CAD build for the part. Positions are in the model's coordinates, mm. A direction names the side the tool comes from. Coordinates: 2 decimals unless noted, no trailing zeros. Order: outer loops, then holes, each group sorted by start corner. A loop starts at its lowest first (then second) coordinate and runs counter-clockwise, first axis right, second up. Notation, with made-up numbers: M 43,83.5 L 62,83.5 A18 cw 62,104.5 Z; hole C 1.5,-7 d6. An arc over 180 degrees is marked long. Write item = value, one per line. Start each with the question number.
Autodesk Inventor part; units mm, degrees
ref_plane "YZ Plane" through (0, 0, 0) normal (1, 0, 0) x (0, 1, 0)
ref_plane "XZ Plane" through (0, 0, 0) normal (0, 1, 0) x (-1, 0, 0)
ref_plane "XY Plane" through (0, 0, 0) normal (0, 0, 1) x (1, 0, 0)
sketch "Sketch1" plane through (0, 0, 0) normal (0, 0, 1) x (1, 0, 0)
  line L0 (0, 0) -> (-132, 0)
  line L1 (-132, 0) -> (-132, -5)
  line L2 (-132, -5) -> (0, -5)
  line L3 (0, -5) -> (0, 0)
  dimension "d0" = 5
  dimension "d1" = 132
extrude "Extrusion1" add sketch "Sketch1" along normal blind 30
sketch "Sketch2" plane through (-132, 0, 0) normal (0, 1, 0) x (1, 0, 0)
  line L0 (0, -30) -> (132, -30)
  line L1 (0, -30) -> (5, -30)
  line L2 (5, -30) -> (5, -15)
  line L3 (5, -15) -> (0, -15)
  line L4 (0, -15) -> (0, -30)
  line L5 (132, -30) -> (127, -30)
  line L6 (127, -30) -> (127, -15)
  line L7 (127, -15) -> (132, -15)
  line L8 (132, -15) -> (132, -30)
  line L9 (0, 0) -> (0, -30)
  line L10 (132, 0) -> (132, -30)
  line L11 (0, 0) -> (132, 0)
  line L12 (132, 0) -> (132, 0)
  line L13 (132, 0) -> (0, 0)
  line L14 (0, 0) -> (0, 0)
  line L15 (0, 0) -> (5, 0)
  line L16 (5, 0) -> (5, -5)
  line L17 (5, -5) -> (0, -5)
  line L18 (0, -5) -> (0, 0)
  line L19 (132, 0) -> (127, 0)
  line L20 (127, 0) -> (127, -5)
  line L21 (127, -5) -> (132, -5)
  line L22 (132, -5) -> (132, 0)
  point P0 (5, -30)
  point P1 (5, 0)
  point P2 (127, 0)
  dimension "d4" = 5
  dimension "d5" = 15
  dimension "d6" = 15
  dimension "d7" = 5
  dimension "d8" = 0
  dimension "d11" = 5
  dimension "d12" = 5
  dimension "d13" = 5
  dimension "d14" = 10
extrude "Extrusion2" cut sketch "Sketch2" against normal blind 10 contours L4 L3 L2 L0 | L6 L7 L8 L0 | L9 L11 L16 L17 | L21 L20 L11 L10
properties part number "FANsuport"
1. Mould opens along X. For faces 1 (the flat face through (-127, -2, 2)), 2 (the flat face through (-5, -2, 23)), 3 (the flat face through (-129, -2, 15)) say: released by +X, released by -X, zero draft, split by the parting line, or undercut.
2. Slice it at B-B (z = 18). Write the cut outline in (x, y), plus the area to 3 significant figures.
3. 3-axis set-ups, long thin cutter, end or side, ignore diameter. For faces 4 (the flat face through (-3, -2, 15)), 5 (the flat face through (-67, -2, 30)), 6 (the flat face through (-3, -2, 5)), 7 (the flat face through (-129, -2, 5)), 8 (the flat face through (-127, -2, 23)): which of +Z, -Z, +X, -X, +Y, -Y reach the whole face in a straight line?
4. Probe L1, parallel to X at y = -0.9, z = 4.75. List the from-to ranges inside material, lowest first.
5. Flat gauge pins, fed straight in: pin 1 (3 mm diameter, centred on x = -38, z = 5.5, fed in from +Y); pin 2 (1.5 mm diameter, centred on x = -130, y = -3.5, fed in from -Z); pin 3 (1.5 mm diameter, centred on y = -2.5, z = 24.5, fed in from +X); pin 4 (1.5 mm diameter, centred on x = -129.5, y = -3, fed in from +Z). Where does each tip first touch, or does it go through?
6. Slice it at A-A (y = -3.95). Write the cut outline in (x, z).
Calculated:
q1.face_1 = released by -X
q1.face_2 = released by +X
q1.face_3 = zero draft
q2.outline = M -127,-5 L -5,-5 L -5,0 L -127,0 Z
q2.area = 610 mm²
q3.face_4 = +Z, +X, +Y, -Y
q3.face_5 = +Z, +X, -X, +Y, -Y
q3.face_6 = -Z, +X, +Y, -Y
q3.face_7 = -Z, -X, +Y, -Y
q3.face_8 = +Z, -X, +Y, -Y
q4.L1 = -127 to -5
q5.pin_1 = 0
q5.pin_2 = 5
q5.pin_3 = -5
q5.pin_4 = 15
q6.outline = M -132,5 L -127,5 L -127,0 L -5,0 L -5,5 L 0,5 L 0,15 L -5,15 L -5,30 L -127,30 L -127,15 L -132,15 Z
